The drawing under review shows one solid part. Ordinate dimensions are in mm from its lowest x, y, z. A direction names the side the tool comes from. Coordinates: 2 decimals unless noted, no trailing zeros. Order: outer loops, then holes, each group sorted by start corner. A loop starts at its lowest first (then second) coordinate and runs counter-clockwise, first axis right, second up.
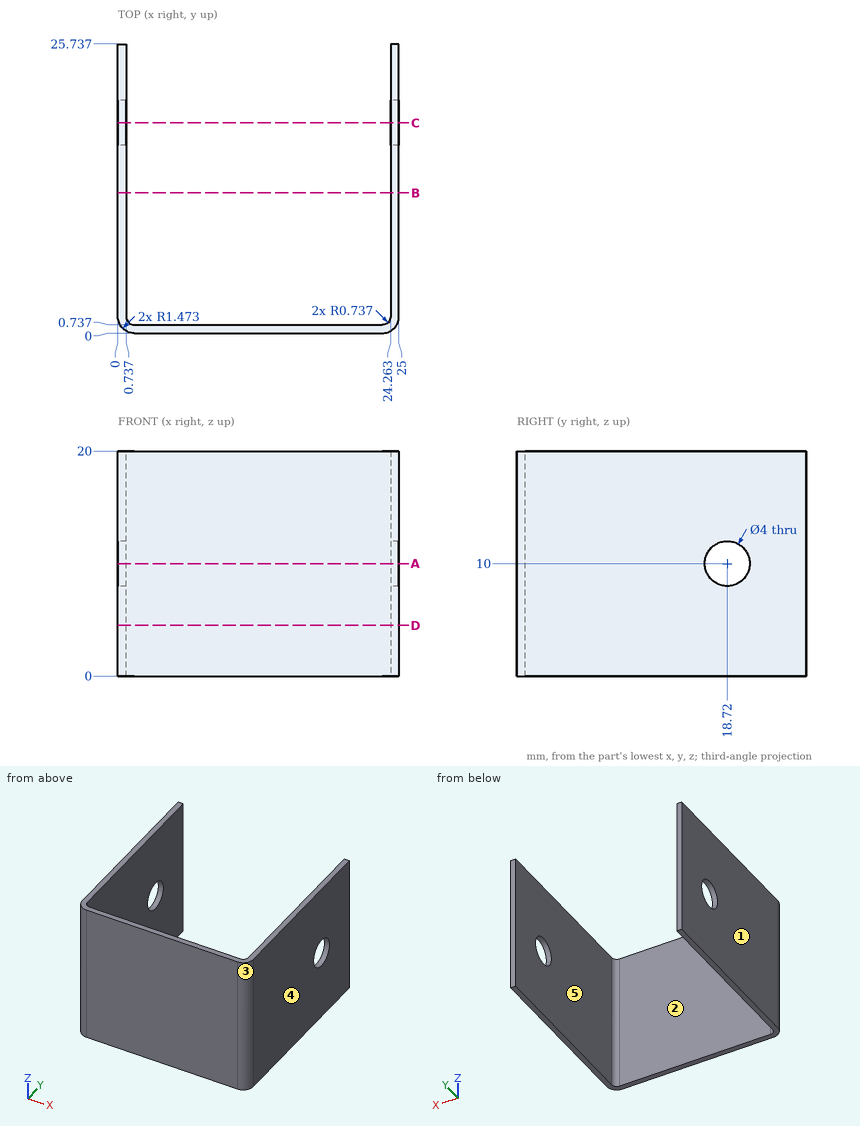
(1) Insertion check: pin 1 Ø2 at (x, z) = (5.5, 12) entering from +Y. The pin has a flat end and moves straight along its axis. Give the tip position at first contact, or say it passes through.
(2) Wall thickness on line 1 (Y direction, x = 24.8, z = 10) (1 decimal); line 2 (X direction, y = 17.25, z = 17.5); line 3 (Y direction, x = 9.5, z = 17): over which ranges is each line inside the solid? List them lowest first.
(3) The part is to be moulded in two halves that separate along X. For the marked faces 1, 2 and 3, say which applies: +X half, -X half, draft (parallel to the pull), parting line (faces both ways), or undercut.
(4) Consider section D-D (z = 4.5). Give the boundary of the cut face in (x, y).
(5) Tool access review of the marked faces 4 and 5: name each direction out of +Z, -Z, +X, -X, +Y, -Y from which nothing blocks a thin tool from reaching the whole face with its end or side.
(6) Consider section B-B (y = 12.5). Give the boundary of the cut face in (x, z).
(7) Consider section A-A (z = 10). Give the boundary of the cut face in (x, y).
(8) Consider section C-C (y = 18.72). Give the boundary of the cut face in (x, z).
Findings:
1. pin 1: stops at y = 0.74
2. line 1: y = 0.7 to 16.7, 20.7 to 25.7
2. line 2: x = 0 to 0.74, 24.26 to 25
2. line 3: y = 0 to 0.74
3. face 1: -X half
3. face 2: undercut
3. face 3: +X half
4. outline: (0, 1.47) arc R1.47 ccw to (1.47, 0) - (23.53, 0) arc R1.47 ccw to (25, 1.47) - (25, 25.74) - (24.26, 25.74) - (24.26, 1.47) arc R0.74 cw to (23.53, 0.74) - (1.47, 0.74) arc R0.74 cw to (0.74, 1.47) - (0.74, 25.74) - (0, 25.74) - close
5. face 4: +Z, -Z, +X, +Y, -Y
5. face 5: +Z, -Z, +Y
6. outline: (0, 0) - (0.74, 0) - (0.74, 20) - (0, 20) - close; (24.26, 0) - (25, 0) - (25, 20) - (24.26, 20) - close
7. outline: (0, 1.47) arc R1.47 ccw to (1.47, 0) - (23.53, 0) arc R1.47 ccw to (25, 1.47) - (25, 16.72) - (24.26, 16.72) - (24.26, 1.47) arc R0.74 cw to (23.53, 0.74) - (1.47, 0.74) arc R0.74 cw to (0.74, 1.47) - (0.74, 16.72) - (0, 16.72) - close; (0, 20.72) - (0.74, 20.72) - (0.74, 25.74) - (0, 25.74) - close; (24.26, 20.72) - (25, 20.72) - (25, 25.74) - (24.26, 25.74) - close
8. outline: (0, 0) - (0.74, 0) - (0.74, 8) - (0, 8) - close; (0, 12) - (0.74, 12) - (0.74, 20) - (0, 20) - close; (24.26, 0) - (25, 0) - (25, 8) - (24.26, 8) - close; (24.26, 12) - (25, 12) - (25, 20) - (24.26, 20) - close
